```python
from build123d import *

# Parameters (mm, degrees)
EXTRUDE_1_DEPTH     = 8
SKETCH_2_R          = 1.5
CUT_EXTRUDE_1_DEPTH = 9
SKETCH_3_R          = 2.5
CUT_EXTRUDE_2_DEPTH = 3


with BuildPart() as part:
    # 草图1 → 凸台-拉伸1 (new body)
    with BuildSketch(Plane.XY):
        Polygon((-16, 0), (0, 4.287187079), (16, 0), (0, -4.287187079), align=None)
    extrude(amount=EXTRUDE_1_DEPTH)

    # 草图2 → 切除-拉伸1 (cut, through all)
    with BuildSketch(Plane(origin=(0, 0, 0), x_dir=(-1, 0, 0), z_dir=(0, 0, -1))):
        with Locations((-3, 0)):
            Circle(SKETCH_2_R)
    extrude(amount=-CUT_EXTRUDE_1_DEPTH, mode=Mode.SUBTRACT)

    # 草图3 → 切除-拉伸2 (cut)
    with BuildSketch(Plane(origin=(0, 0, 0), x_dir=(-1, 0, 0), z_dir=(0, 0, -1))):
        with Locations((-3, 0)):
            Circle(SKETCH_3_R)
    extrude(amount=-CUT_EXTRUDE_2_DEPTH, mode=Mode.SUBTRACT)


solid = part.part
```
The listing builds one solid part. Answer for the finished solid, in the listing's coordinates (mm). A direction names the side the tool comes from. Coordinates: 2 decimals unless noted, no trailing zeros. Write each loop counter-clockwise with the first axis right and the second up, starting at its lowest first coordinate (ties: lowest second). Pieces come first, ordered by that corner, then holes. Notation, with made-up numbers: (-31.75, -34.75) - (-7.75, -34.75) arc R25 cw to (-7.75, -7.75) - close; hole circle Ø2 at (85.25, 76.5). An arc over 180 degrees is marked (long way). Return JSON: item names as keys, results as strings. Group by question number.
1. A cutting plane is placed at D-D, the plane z = 4.5. Determine the outline of the cut face in (x, y), plus the area to 3 significant figures.
2. Which of the six approach directions +Z, -Z, +X, -X, +Y, -Y give full straight-line access (tool end or side, diameter ignored) to faces 4 (the cylindrical face through (0.615, 0.751, 1.479)), 5 (the flat face through (-7.888, -2.174, 3.944))?
3. Determine the mould class of faces 1 (the flat face through (0, 0, 0)), 2 (the cylindrical face through (1.57, 0.45, 5.46)), 3 (the flat face through (-8.112, 2.114, 3.944)) for opening direction X: released by +X, released by -X, zero draft, split by the parting line, or undercut.
4. Given pin 1 (1.5 mm diameter, centred on x = 9, y = 3.5, fed in from +Z), flat-ended and moving along its own axis, determine where the tip first touches the part or whether it passes through.
5. A cutting plane is placed at B-B, the plane y = 0.75. Determine the outline of the cut face in (x, z).
6. Straight lines are drawn through the part: L1, parallel to Y at x = 3, z = 5.8; L2, parallel to Z at x = 1.5, y = -1.25; L3, parallel to Y at x = 2, z = 6. For each, find the intervals that lie inside material, in ascending order.
7. A cutting plane is placed at A-A, the plane z = 1.25. Determine the outline of the cut face in (x, y).
8. A cutting plane is placed at C-C, the plane x = 3. Determine the outline of the cut face in (y, z), plus the area to 3 significant figures.
Ans:
{
 "1": {"outline": "(-16, 0) - (0, -4.29) - (16, 0) - (0, 4.29) - close; hole circle Ø3 at (3, 0)", "area": "130 mm²"},
 "2": {"face 4": "-Z", "face 5": "+Z, -Z, -X, -Y"},
 "3": {"face 1": "zero draft", "face 2": "undercut", "face 3": "released by -X"},
 "4": {"pin 1": "through"},
 "5": {"outline": "(-13.2, 0) - (0.62, 0) - (0.62, 3) - (1.7, 3) - (1.7, 8) - (-13.2, 8) - close; (4.3, 3) - (5.38, 3) - (5.38, 0) - (13.2, 0) - (13.2, 8) - (4.3, 8) - close"},
 "6": {"L1": "-3.48 to -1.5, 1.5 to 3.48", "L2": "3 to 8", "L3": "-3.75 to -1.12, 1.12 to 3.75"},
 "7": {"outline": "(-16, 0) - (0, -4.29) - (16, 0) - (0, 4.29) - close; hole circle Ø5 at (3, 0)"},
 "8": {"outline": "(-3.48, 0) - (-2.5, 0) - (-2.5, 3) - (-1.5, 3) - (-1.5, 8) - (-3.48, 8) - close; (1.5, 3) - (2.5, 3) - (2.5, 0) - (3.48, 0) - (3.48, 8) - (1.5, 8) - close", "area": "25.7 mm²"}
}
